Can you work these out from the model? Positions are in its coordinate system, mm. A direction names the side the tool comes from. Coordinates: 2 decimals unless noted, no trailing zeros. Write each loop counter-clockwise with the first axis right and the second up, starting at its lowest first coordinate (ties: lowest second). Pieces come first, ordered by that corner, then holes.
Autodesk Inventor part; units mm, degrees
ref_plane "YZ Plane" through (0, 0, 0) normal (1, 0, 0) x (0, 1, 0)
ref_plane "XZ Plane" through (0, 0, 0) normal (0, 1, 0) x (-1, 0, 0)
ref_plane "XY Plane" through (0, 0, 0) normal (0, 0, 1) x (1, 0, 0)
sketch "Эскиз1" plane through (0, 0, 0) normal (0, 1, 0) x (-1, 0, 0)
  line L0 (-12, 12) -> (12, 12) construction
  line L1 (12, 12) -> (12, -12) construction
  line L2 (12, -12) -> (-12, -12) construction
  line L3 (-12, -12) -> (-12, 12) construction
  line L4 (-12, 12) -> (12, -12) construction
  line L5 (12, 12) -> (-12, -12) construction
  line L6 (-15, -15) -> (15, -15)
  line L7 (15, -15) -> (15, 15)
  line L8 (15, 15) -> (-15, 15)
  line L9 (-15, 15) -> (-15, -15)
  line L10 (-15, -15) -> (15, 15) construction
  line L11 (15, -15) -> (-15, 15) construction
  circle A0 centre (0, 0) radius 14
  circle A1 centre (-12, -12) radius 1.5
  circle A2 centre (-12, 12) radius 1.5
  circle A3 centre (12, 12) radius 1.5
  circle A4 centre (12, -12) radius 1.5
  dimension "d0" = 24
  dimension "d1" = 24
  dimension "d2" = 30
  dimension "d3" = 30
  dimension "d4" = 28
  dimension "d8" = 3
  dimension "d9" = 3
  dimension "d10" = 3
  dimension "d11" = 3
extrude "Выдавливание1" add sketch "Эскиз1" along normal blind 2
sketch "Эскиз2" plane through (0, 0, 0) normal (0, -1, 0) x (1, 0, 0)
  circle A0 centre (0, 0) radius 14
  circle A1 centre (-12, -12) radius 1.5
  circle A2 centre (-12, 12) radius 1.5
  circle A3 centre (12, 12) radius 1.5
  circle A4 centre (12, -12) radius 1.5
  circle A5 centre (0, 0) radius 15
  circle A6 centre (-12, -12) radius 2.5
  circle A7 centre (-12, 12) radius 2.5
  circle A8 centre (12, 12) radius 2.5
  circle A9 centre (12, -12) radius 2.5
  dimension "d14" = 5
  dimension "d15" = 5
  dimension "d16" = 5
  dimension "d17" = 5
extrude "Выдавливание2" add sketch "Эскиз2" along normal blind 8
sketch "Эскиз4" plane through (0, -8, 0) normal (0, -1, 0) x (1, 0, 0)
  circle A0 centre (12, 12) radius 1.5
  circle A1 centre (-12, -12) radius 1.5
  circle A2 centre (-12, 12) radius 1.5
  circle A3 centre (12, -12) radius 1.5
  circle A4 centre (0, 0) radius 14
  arc A5 (11.5789, -9.5357) -> (11.5789, 9.5357) centre (0, 0) ccw
  line L0 (-15, 15) -> (15, 15)
  line L1 (15, 15) -> (15, -15)
  line L2 (15, -15) -> (-15, -15)
  line L3 (-15, -15) -> (-15, 15)
  circle A6 centre (0, 0) radius 7.5
  line L4 (0, 0) -> (0, 15) construction
  line L5 (0, 0) -> (-12.1244, -7) construction
  line L6 (0, 0) -> (12.1244, -7) construction
  line L7 (-0.75, 6.7531) -> (0.75, 6.7531)
  line L8 (0.75, 6.7531) -> (0.75, 14.2469)
  line L9 (0.75, 14.2469) -> (-0.75, 14.2469)
  line L10 (-0.75, 14.2469) -> (-0.75, 6.7531)
  line L11 (-0.75, 6.7531) -> (0.75, 14.2469) construction
  line L12 (0.75, 6.7531) -> (-0.75, 14.2469) construction
  line L13 (-5.565, -4.079) -> (-6.315, -2.7799)
  line L14 (-6.315, -2.7799) -> (-12.8048, -6.5268)
  line L15 (-12.8048, -6.5268) -> (-12.0548, -7.8259)
  line L16 (-12.0548, -7.8259) -> (-5.565, -4.079)
  line L17 (-5.565, -4.079) -> (-12.8048, -6.5268) construction
  line L18 (-6.315, -2.7799) -> (-12.0548, -7.8259) construction
  line L19 (6.315, -2.7799) -> (5.565, -4.079)
  line L20 (5.565, -4.079) -> (12.0548, -7.8259)
  line L21 (12.0548, -7.8259) -> (12.8048, -6.5268)
  line L22 (12.8048, -6.5268) -> (6.315, -2.7799)
  line L23 (6.315, -2.7799) -> (12.0548, -7.8259) construction
  line L24 (5.565, -4.079) -> (12.8048, -6.5268) construction
  point P0 (0, 10.5)
  point P1 (-9.1849, -5.3029)
  point P2 (9.1849, -5.3029)
  dimension "d22" = 15
  dimension "d23" = 120
  dimension "d24" = 120
  dimension "d25" = 1.5
  dimension "d26" = 1.5
  dimension "d27" = 1.5
extrude "Выдавливание4" add sketch "Эскиз4" along normal blind 2 contours L8 A6 L10 A4 | A4 L10 L9 L8 | L22 L21 L20 A4 | A4 L20 A6 L22 | L8 L7 L10 A6 | A6 L22 L19 L20 L16 L13 L14 L10 L7 L8 | A6 L20 L19 L22 | L14 A6 L16 A4 | A4 L16 L15 L14 | L14 L13 L16 A6 | L0 L1 L2 L3
fillet "Сопряжение1" radius 2 8 edges at (-15, -9, -15) (15, -9, -15) (15, 1, -15) (-15, 1, -15) (-15, 1, 15) (-15, -9, 15) (15, 1, 15) (15, -9, 15)
properties part number "Cooler"
1. If we section it at A-A, the plane y = -8.5: List the corners of the cut face in (x, z) for me.
2. If I drill on L1, parallel to Z at x = 4.5, y = -8.5; L2, parallel to X at y = -3.75, z = -12, over which ranges is the centre line in solid material (lowest first)?
3. I'm going to push a flat-ended pin straight in: P1, Ø2.5, axis at x = -12, z = -12, coming from the +Y side. Where does the tip first touch, or does it pass through?
4. If we section it at B-B, the plane z = 4.5: List the corners of the cut face in (x, y) for me, plus the area to 3 significant figures.
5. If we section it at D-D, the plane z = -10: List the corners of the cut face in (x, y) for me.
6. We'd pull the mould along Y, two halves only. Please class faces 1 (the face through (0, -4, -15)), 2 (the face through (6.445, -8.986, 3.836)): released by +Y, released by -Y, zero draft, split by the parting line, or undercut.
7. If we section it at C-C, the plane y = 1.25: List the corners of the cut face in (x, z) for me, plus the area to 3 significant figures.
8. Which directions (+Z, -Z, +X, -X, +Y, -Y) give clear straight access to the entire face, cutting with the end or side of a thin tool? Please do faces 3 (the face through (13, 0, 9)), 4 (the face through (15, 1, 0)), 5 (the face through (-8.949, -8.986, -6.033)).
Answers:
1. outline: (-15, -13) arc R2 ccw to (-13, -15) - (13, -15) arc R2 ccw to (15, -13) - (15, 13) arc R2 ccw to (13, 15) - (-13, 15) arc R2 ccw to (-15, 13) - close; hole circle Ø3 at (-12, -12); hole circle Ø3 at (-12, 12); hole (-12.48, -6.34) - (-6.84, -3.08) arc R7.5 cw to (-0.75, 7.46) - (-0.75, 13.98) arc R14 ccw to start; hole (-11.73, -7.64) arc R14 ccw to (11.73, -7.64) - (6.09, -4.38) arc R7.5 cw to (-6.09, -4.38) - close; hole (0.75, 7.46) arc R7.5 cw to (6.84, -3.08) - (12.48, -6.34) arc R14 ccw to (0.75, 13.98) - close; hole circle Ø3 at (12, -12); hole circle Ø3 at (12, 12)
2. L1: z = -15 to -13.26, -6 to 6, 13.26 to 15
2. L2: x = -14.5 to -13.5, -10.5 to -9.5, -9 to -7.21, 7.21 to 9, 9.5 to 10.5, 13.5 to 14.5
3. P1: passes through
4. outline: (-15, -10) - (-13.26, -10) - (-13.26, 2) - (-15, 2) - (-15, 0) - (-14.31, 0) - (-14.31, -8) - (-15, -8) - close; (-6, -10) - (6, -10) - (6, -8) - (-6, -8) - close; (13.26, -10) - (15, -10) - (15, -8) - (14.31, -8) - (14.31, 0) - (15, 0) - (15, 2) - (13.26, 2) - close
4. area: 54.8 mm2
5. outline: (-15, -10) - (-9.8, -10) - (-9.8, 2) - (-15, 2) - (-15, 0) - (-13.5, 0) - (-13.5, -8) - (-15, -8) - close; (9.8, -10) - (15, -10) - (15, -8) - (13.5, -8) - (13.5, 0) - (15, 0) - (15, 2) - (9.8, 2) - close
6. face 1: undercut
6. face 2: zero draft
7. outline: (-15, -13) arc R2 ccw to (-13, -15) - (13, -15) arc R2 ccw to (15, -13) - (15, 13) arc R2 ccw to (13, 15) - (-13, 15) arc R2 ccw to (-15, 13) - close; hole circle Ø28 at (0, 0); hole circle Ø3 at (-12, -12); hole circle Ø3 at (-12, 12); hole circle Ø3 at (12, -12); hole circle Ø3 at (12, 12)
7. area: 253 mm2
8. face 3: none
8. face 4: +Z, -Z, +X, +Y, -Y
8. face 5: +Y, -Y
